Can you work these out from the drawing? Everything is in mm from the part's minimum corner. Coordinates: 2 decimals unless noted, no trailing zeros. Write each loop counter-clockwise with the first axis right and the second up, starting at its lowest first coordinate (ties: lowest second). Pieces come first, ordered by that corner, then holes. Notation, with made-up numbers: M 75.25,26.5 L 121.25,26.5 A20 cw 121.25,37.5 Z; hole C 27.5,21.25 d1. An arc over 180 degrees is marked long. Write item = value, one per line.
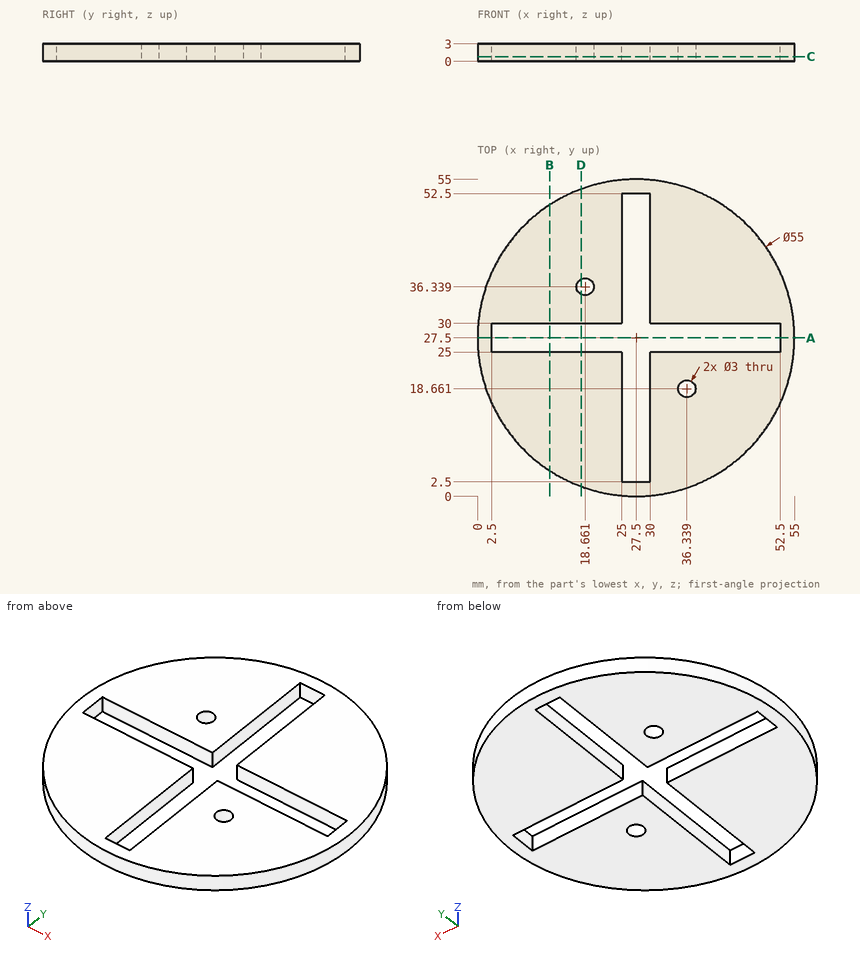
Item 1: Imagine slicing it at D-D (x = 18). Write out the boundary of the cut face in (y, z) (1 decimal), and give its area (3 significant figures).
Numbers:
outline = M 1.7,0 L 25,0 L 25,3 L 1.7,3 Z; M 30,0 L 35,0 L 35,3 L 30,3 Z; M 37.7,0 L 53.3,0 L 53.3,3 L 37.7,3 Z
area = 132 mm²
Item 2: Imagine slicing it at B-B (x = 12.5). Write out the boundary of the cut face in (y, z), and give its area (3 significant figures).
Numbers:
outline = M 4.45,0 L 25,0 L 25,3 L 4.45,3 Z; M 30,0 L 50.55,0 L 50.55,3 L 30,3 Z
area = 123 mm²
Item 3: If I drill on line 1 along Y through (x, z) = (28, 1.1); line 2 along Y through (x, z) = (36, 0.75), over which ranges is the centre line in solid material (lowest first)?
Numbers:
line_1 = 0 to 2.5, 52.5 to 55
line_2 = 1.35 to 17.2, 20.12 to 25, 30 to 53.65
Item 4: Imagine slicing it at C-C (z = 0.8). Write out the boundary of the cut face in (x, y), and give its area (3 significant figures).
Numbers:
outline = C 27.5,27.5 d55; hole M 2.5,25 L 25,25 L 25,2.5 L 30,2.5 L 30,25 L 52.5,25 L 52.5,30 L 30,30 L 30,52.5 L 25,52.5 L 25,30 L 2.5,30 Z; hole C 18.66,36.34 d3; hole C 36.34,18.66 d3
area = 1,890 mm²
Item 5: I'm going to push flat-ended pins straight in: P1, Ø2.5, axis at x = 18.66, y = 36.34, coming from the -Z side; P2, Ø4, axis at x = 36.34, y = 18.66, coming from the +Z side; P3, Ø1.5, axis at x = 30.5, z = 2, coming from the -Y side; P4, Ø1.5, axis at y = 31.5, z = 2, coming from the -X side. Where does each tip first touch, or does it pass through?
Numbers:
P1 = through
P2 = 3
P3 = 0.09
P4 = 0.19
Item 6: Imagine slicing it at A-A (y = 27.5). Write out the boundary of the cut face in (x, z).
Numbers:
outline = M 0,0 L 2.5,0 L 2.5,3 L 0,3 Z; M 52.5,0 L 55,0 L 55,3 L 52.5,3 Z
